Geometry: final body of the model. Coordinates: model frame, mm. Face numbers are marked on the shaded views. A direction names the side the tool comes from. Coordinates: 2 decimals unless noted, no trailing zeros. Write each loop counter-clockwise with the first axis right and the second up, starting at its lowest first coordinate (ties: lowest second). Pieces come first, ordered by that corner, then holes. Notation, with made-up numbers: (54.25, 23) -> (103.25, 23) arc R26 ccw to (103.25, 54) -> close; hole circle Ø8 at (24, 81.5). An arc over 180 degrees is marked (long way). Answer as a JSON object with one key per item and string values. Group by question number.
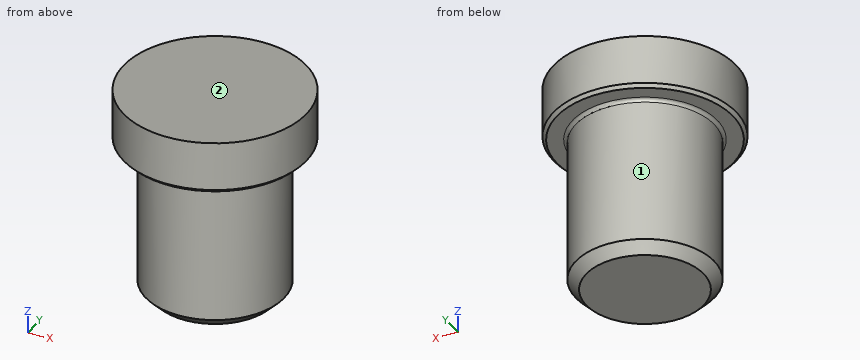
```python
from build123d import *

# Parameters (mm, degrees)
F2_R    = 1.5875
F3_SIZE = 1.5875
F4_SIZE = 5.08


with BuildPart() as f1:
    # F0 (on Front) → F1 (revolve)
    with BuildSketch(Plane.XZ):
        Polygon((0, 50.8), (0, -50.8), (33.655, -50.8), (33.655, 25.4), (44.45, 25.4), (44.45, 50.8), align=None)
    revolve(axis=Axis((0, 0, 0), (0, 0, 1)))

    # F2
    f2_edges = [f1.edges().sort_by_distance(p)[0] for p in [
        (-33.655, 0, 25.4),
    ]]
    fillet(f2_edges, radius=F2_R)

    # F3
    f3_edges = [f1.edges().sort_by_distance(p)[0] for p in [
        (-44.45, 0, 25.4),
    ]]
    chamfer(f3_edges, length=F3_SIZE)

    # F4
    f4_edges = [f1.edges().sort_by_distance(p)[0] for p in [
        (-33.655, 0, -50.8),
    ]]
    chamfer(f4_edges, length=F4_SIZE)


solid = f1.part
```
Item 1: Set-up query: the marked faces 1 and 2. Return all of +Z, -Z, +X, -X, +Y, -Y with unobstructed straight access to the full face (end or side cutting, diameter ignored); none if empty.
Item 2: Contact query for flat-ended pins moving along their axis: pin 1 (12 mm diameter, centred on x = -3.5, z = 18.5, fed in from +Y); pin 2 (2 mm diameter, centred on y = -8, z = -11, fed in from -X); pin 3 (5 mm diameter, centred on x = 33, z = 36, fed in from +Y) (3 decimals). Output: stop coordinate, or through.
Item 3: Section D-D on z = -10.5. Output: boundary loops of the cut face in (x, y) (3 decimals), then the cut area to 3 significant figures.
Item 4: Ray query, L1, parallel to Z at x = 19, y = -33.5; L2, parallel to Y at x = -9.5, z = 10; L3, parallel to X at y = -0.5, z = 2.5. Return the intervals inside material, ascending. Write a range as [from, to].
Item 5: Section C-C on z = 41. Output: boundary loops of the cut face in (x, y), then the cut area to 3 significant figures.
Answer sheet:
{
 "1": {"face 1": "-Z", "face 2": "+Z, +X, -X, +Y, -Y"},
 "2": {"pin 1": "stops at y = 33.68", "pin 2": "stops at x = -32.92", "pin 3": "stops at y = 32.335"},
 "3": {"outline": "circle Ø67.31 at (0, 0)", "area": "3,560 mm^2"},
 "4": {"L1": "z = [25.4, 50.8]", "L2": "y = [-32.29, 32.29]", "L3": "x = [-33.65, 33.65]"},
 "5": {"outline": "circle Ø88.9 at (0, 0)", "area": "6,210 mm^2"}
}
